Build history of the part. All positions in model axes, mm. Face numbers are marked on the shaded views. Give positions to 0.01 mm unless a question says otherwise; leave off trailing zeros. Order: outer loops, then holes, each group sorted by start corner. A loop starts at its lowest first (then second) coordinate and runs counter-clockwise, first axis right, second up. Notation, with made-up numbers: (20.5, 84.5) - (25.5, 84.5) arc R31 cw to (25.5, 118.5) - close; hole circle Ø9 at (-25, 17.5). An arc over 180 degrees is marked (long way). Use a Markdown table: item, result.
from build123d import *

# Parameters (mm, degrees)
F0_W     = 88.9
F0_H     = 88.9
F1_DEPTH = 6.35
F2_W     = 76.2
F2_H     = 76.2
F3_DEPTH = 6.35
F4_W     = 6.35
F4_H     = 63.5
F5_DEPTH = 19.05
F6_R     = 7.56699
F7_DEPTH = 25.4


with BuildPart() as f1:
    # F0 (on Top) → F1 (new body)
    with BuildSketch(Plane.XY):
        Rectangle(F0_W, F0_H)
    extrude(amount=F1_DEPTH)

    # F2 (on face) → F3 (join)
    with BuildSketch(Plane(origin=(0, 0, 0), x_dir=(1, 0, 0), z_dir=(0, 0, -1))):
        Rectangle(F2_W, F2_H)
    extrude(amount=F3_DEPTH)

    # F4 (on face) → F5 (join)
    with BuildSketch(Plane.XY.offset(6.35)):
        Rectangle(F4_W, F4_H)
    extrude(amount=F5_DEPTH)

    # F6 (on face) → F7 (cut)
    with BuildSketch(Plane.XY.offset(6.35)):
        with Locations((26.67, -26.67)):
            Circle(F6_R)
    extrude(amount=-F7_DEPTH, mode=Mode.SUBTRACT)


solid = f1.part
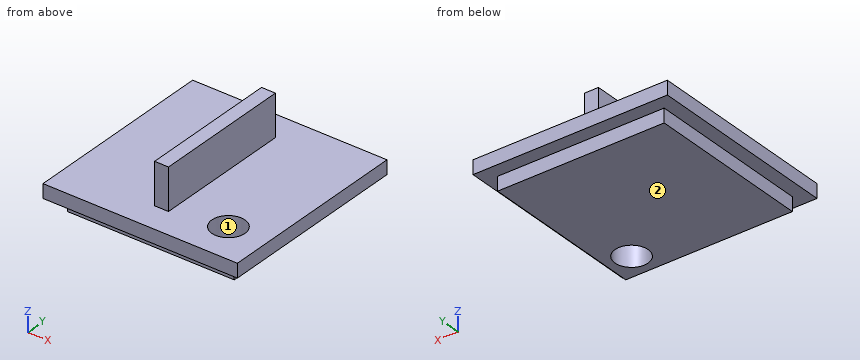
1) Slice it at D-D (y = 29). Write the cut outline in (x, z) (3 decimals), and give its area (3 significant figures).
Computed:
| item | result |
|---|---|
| outline | (-44.45, 0) - (-38.1, 0) - (-38.1, -6.35) - (38.1, -6.35) - (38.1, 0) - (44.45, 0) - (44.45, 6.35) - (3.175, 6.35) - (3.175, 25.4) - (-3.175, 25.4) - (-3.175, 6.35) - (-44.45, 6.35) - close |
| area | 1,170 mm² |
2) Slice it at C-C (z = -3.5). Write the cut outline in (x, y).
Computed:
| item | result |
|---|---|
| outline | (-38.1, -38.1) - (38.1, -38.1) - (38.1, 38.1) - (-38.1, 38.1) - close; hole circle Ø15.13 at (26.67, -26.67) |
3) Slice it at B-B (x = 26.67). Write the cut outline in (y, z).
Computed:
| item | result |
|---|---|
| outline | (-44.45, 0) - (-38.1, 0) - (-38.1, -6.35) - (-34.24, -6.35) - (-34.24, 6.35) - (-44.45, 6.35) - close; (-19.1, -6.35) - (38.1, -6.35) - (38.1, 0) - (44.45, 0) - (44.45, 6.35) - (-19.1, 6.35) - close |
4) Wall check: line 1 (Y direction, x = 26.67, z = -3); line 2 (Y direction, x = 26.67, z = 2.5); line 3 (X direction, y = 6.5, z = 22.5) (3 decimals). Give the ranges that are in metal, low to high. Write a range as from..to.
Computed:
| item | result |
|---|---|
| line 1 | y = -38.1..-34.24, -19.1..38.1 |
| line 2 | y = -44.45..-34.24, -19.1..44.45 |
| line 3 | x = -3.175..3.175 |
5) Slice it at A-A (y = -26.67). Write the cut outline in (x, z) (3 decimals).
Computed:
| item | result |
|---|---|
| outline | (-44.45, 0) - (-38.1, 0) - (-38.1, -6.35) - (19.103, -6.35) - (19.103, 6.35) - (3.175, 6.35) - (3.175, 25.4) - (-3.175, 25.4) - (-3.175, 6.35) - (-44.45, 6.35) - close; (34.237, -6.35) - (38.1, -6.35) - (38.1, 0) - (44.45, 0) - (44.45, 6.35) - (34.237, 6.35) - close |
6) Two-plate mould, pull along Y, no slides. Class the marked faces 1 and 2: +Y half, -Y half, draft (parallel to the pull), parting line (faces both ways), or undercut.
Computed:
| item | result |
|---|---|
| face 1 | undercut |
| face 2 | draft |
7) Pin check, flat tips, straight feed: P1, Ø7, axis at x = 1, z = 19.5, coming from the -Y side; P2, Ø6, axis at x = 16.5, y = 19, coming from the +Z side; P3, Ø5, axis at x = 1, z = 16, coming from the +Y side. Stop position of each tip, or through.
Computed:
| item | result |
|---|---|
| P1 | stops at y = -31.75 |
| P2 | stops at z = 6.35 |
| P3 | stops at y = 31.75 |
